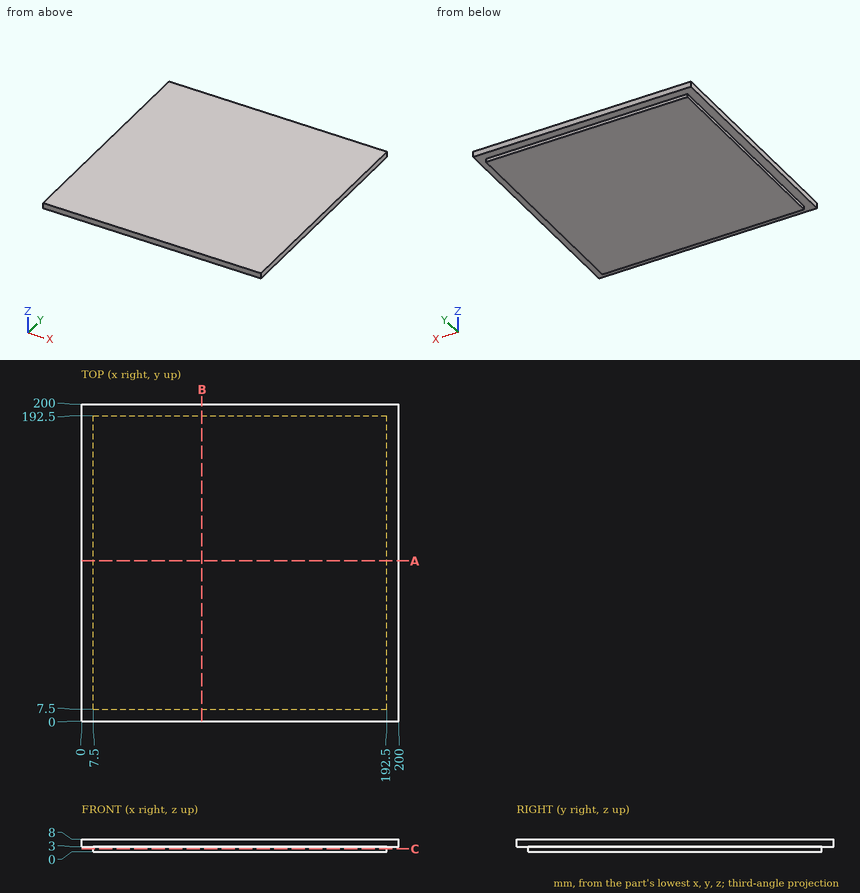
Geometry check sheet. Reference: drawing and pictorial views, mm from the part's lowest x, y, z. Coordinates: 2 decimals unless noted, no trailing zeros. Write each loop counter-clockwise with the first axis right and the second up, starting at its lowest first coordinate (ties: lowest second). Pieces come first, ordered by that corner, then holes. Notation, with made-up numbers: (-35, -7) -> (24, -7) arc R12 ccw to (24, 2) -> close; hole circle Ø1 at (55, 32.25). An arc over 180 degrees is marked (long way). Use a Markdown table: item, result.
1. Scan line: line 1 along X through (y, z) = (127.5, 2). Record every from-to range of solid material in increasing order.
Reported:
| item | result |
|---|---|
| line 1 | x = 7.5 to 192.5 |
2. Sectioned sample at C-C (z = 1.75). Enter the section's corners in (x, y).
Reported:
| item | result |
|---|---|
| outline | (7.5, 7.5) -> (192.5, 7.5) -> (192.5, 192.5) -> (7.5, 192.5) -> close |
3. Sectioned sample at A-A (y = 101). Enter the section's corners in (x, z).
Reported:
| item | result |
|---|---|
| outline | (0, 3) -> (7.5, 3) -> (7.5, 0) -> (192.5, 0) -> (192.5, 3) -> (200, 3) -> (200, 8) -> (0, 8) -> close |
4. Go/stop test with flat-tipped pins: pin 1 Ø2.5 at (y, z) = (76.5, 1) entering from -X; pin 2 Ø0.9 at (x, z) = (99, 2) entering from +Y; pin 3 Ø0.9 at (y, z) = (143, 1) entering from +X. Record where each tip stops, or that it passes through.
Reported:
| item | result |
|---|---|
| pin 1 | stops at x = 7.5 |
| pin 2 | stops at y = 192.5 |
| pin 3 | stops at x = 192.5 |
